CAD build for the part. Positions are in the model's coordinates, mm. A direction names the side the tool comes from. Coordinates: 2 decimals unless noted, no trailing zeros. Write each loop counter-clockwise with the first axis right and the second up, starting at its lowest first coordinate (ties: lowest second). Pieces come first, ordered by that corner, then holes. Notation, with made-up numbers: M 56.5,83 L 98.5,83 A16 ccw 98.5,90 Z; hole C -2,21 d2. An arc over 180 degrees is marked long. Put each result on its own line as item: value. Start each with the question number.
```python
from build123d import *

# Parameters (mm, degrees)
F0_W     = 89.4640423357
F0_H     = 90.7079130411
F1_DEPTH = 25.4
F2_W     = 89.4640423357
F2_H     = 21.721240133
F3_DEPTH = 101.6
F4_W     = 17.7147258073
F4_H     = 18.108388409
F4_W_2   = 18.5020421632
F4_H_2   = 17.3210632056
F4_W_3   = 12.5971408561
F4_H_3   = 18.1083856151
F4_W_4   = 16.9274024665
F5_DEPTH = 76.2
F6_R     = 5.08


with BuildPart() as f1:
    # F0 (on Top) → F1 (new body)
    with BuildSketch(Plane.XY):
        with Locations((-10.2659445256, -7.1802102029)):
            Rectangle(F0_W, F0_H)
    extrude(amount=F1_DEPTH)

    # F2 (on face) → F3 (join)
    with BuildSketch(Plane.XY.offset(25.4)):
        with Locations((-10.2659445256, 27.3131262511)):
            Rectangle(F2_W, F2_H)
    extrude(amount=F3_DEPTH)

    # F4 (on face) → F5 (join)
    with BuildSketch(Plane(origin=(0, 0, 0), x_dir=(1, 0, 0), z_dir=(0, 0, -1))):
        with Locations((-38.7079184875, 35.0316995755)):
            Rectangle(F4_W, F4_H)
        with Locations((13.6489381548, 36.21267993)):
            Rectangle(F4_W_2, F4_H_2)
        with Locations((13.8457692228, -19.687120337)):
            Rectangle(F4_W_3, F4_H_3)
        with Locations((-36.7396157235, -20.8681025542)):
            Rectangle(F4_W_4, F4_H_3)
    extrude(amount=F5_DEPTH)

    # F6
    f6_edges = [f1.edges().sort_by_distance(p)[0] for p in [
        (34.466077, 16.452506, 76.2),
        (-54.997966, 16.452506, 76.2),
    ]]
    fillet(f6_edges, radius=F6_R)


solid = f1.part
```
(1) Drop flat-ended pins along their axis: pin 1 (14.5 mm diameter, centred on y = -31.5, z = -46, fed in from +X); pin 2 (13.5 mm diameter, centred on x = -38, z = -38.5, fed in from +Y); pin 3 (14.5 mm diameter, centred on y = -33, z = -52.5, fed in from -X). Give the stop position or say it passes through.
(2) Slice it at C-C, the plane y = -24. Write the cut outline in (x, z).
(3) Drill centre lines: line 1 (Y direction, x = 20, z = -61); line 2 (Z direction, x = 16, y = -2); line 3 (Z direction, x = -33, y = -43). Where is each one in solid material? Low to high. Write a range as [from, to].
(4) Which spindle directions (+Z, -Z, +X, -X, +Y, -Y) get a long thin tool onto all of the face, cutting with end or side? Do faces 1 (the face through (-37, 11.814, -38)), 2 (the face through (-37, 29.922, -38)), 3 (the face through (14, -44.873, -38)). Say none if no direction does.
(5) Slice it at A-A, the plane z = -18. Write the cut outline in (x, y), then the cut area to 3 significant figures.
(6) Two-plate mould, pull along X, no slides. Class faces 4 (the face through (22.9, -36, -38)), 5 (the face through (-11, -23, 25.4)), 6 (the face through (-28.276, 21, -38)), 7 (the face through (4.398, -36, -38)): +X half, -X half, draft (parallel to the pull), parting line (faces both ways), or undercut.
(7) Slice it at B-B, the plane x = -34.5. Write the cut outline in (y, z), then the cut area to 3 significant figures.
(8) Slice it at D-D, the plane x = -11. Write the cut outline in (y, z).
Result set:
1. pin 1: stops at x = 22.9
1. pin 2: stops at y = 29.92
1. pin 3: stops at x = -47.57
2. outline: M -55,0 L 34.47,0 L 34.47,25.4 L -55,25.4 Z
3. line 1: y = [-44.87, -27.55], [10.63, 28.74]
3. line 2: z = [0, 25.4]
3. line 3: z = [-76.2, 25.4]
4. face 1: -Z, -X
4. face 2: -Z, +X, -X, +Y
4. face 3: -Z, +X, -X, -Y
5. outline: M -47.57,-44.09 L -29.85,-44.09 L -29.85,-25.98 L -47.57,-25.98 Z; M -45.2,11.81 L -28.28,11.81 L -28.28,29.92 L -45.2,29.92 Z; M 4.4,-44.87 L 22.9,-44.87 L 22.9,-27.55 L 4.4,-27.55 Z; M 7.55,10.63 L 20.14,10.63 L 20.14,28.74 L 7.55,28.74 Z
5. area: 1,180 mm^2
6. face 4: +X half
6. face 5: draft
6. face 6: undercut
6. face 7: undercut
7. outline: M -52.53,0 L -44.09,0 L -44.09,-76.2 L -25.98,-76.2 L -25.98,0 L 11.81,0 L 11.81,-76.2 L 29.92,-76.2 L 29.92,0 L 38.17,0 L 38.17,127 L 16.45,127 L 16.45,25.4 L -52.53,25.4 Z
7. area: 7,270 mm^2
8. outline: M -52.53,0 L 38.17,0 L 38.17,127 L 16.45,127 L 16.45,25.4 L -52.53,25.4 Z
